Check sheet for the modelled part. Datum: model origin and axes. Units: mm. Face numbers are marked on the shaded views. Round coordinates to 2 decimals unless told otherwise and drop trailing zeros. Write each loop counter-clockwise with the first axis right and the second up, starting at its lowest first coordinate (ties: lowest second). Pieces come first, ordered by that corner, then holes.
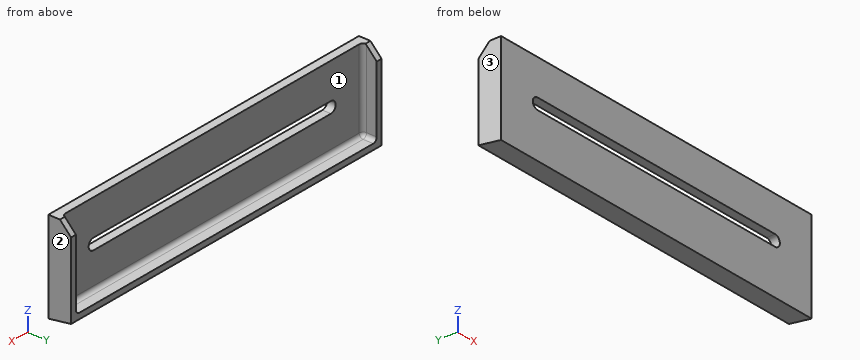
from build123d import *

# Parameters (mm, degrees)
SKETCH1_W           = 101.6
SKETCH1_H           = 25.4
BOSS_EXTRUDE1_DEPTH = 6.35
CUT_EXTRUDE2_DEPTH  = 101.6
SKETCH4_W           = 98.425
SKETCH4_H           = 22.79142
CUT_EXTRUDE3_DEPTH  = 3.96748
CUT_EXTRUDE6_DEPTH  = 2.54
CUT_EXTRUDE7_DEPTH  = 1.5875
CUT_EXTRUDE8_DEPTH  = 1.5875
FILLET1_R           = 1.12268


with BuildPart() as part:
    # Sketch1 → Boss-Extrude1 (new body)
    with BuildSketch(Plane(origin=(0, 0, 0), x_dir=(1, 0, 0), z_dir=(0, 1, 0))):
        Rectangle(SKETCH1_W, SKETCH1_H)
    extrude(amount=BOSS_EXTRUDE1_DEPTH)

    # Sketch2 → Cut-Extrude2 (cut)
    with BuildSketch(Plane.ZY.offset(50.8)):
        Polygon((-12.7, 0), (-11.67892, 6.35), (-12.7, 6.35), align=None)
    extrude(amount=-CUT_EXTRUDE2_DEPTH, mode=Mode.SUBTRACT)

    # Sketch4 → Cut-Extrude3 (cut)
    with BuildSketch(Plane(origin=(0, 6.35, 0), x_dir=(1, 0, 0), z_dir=(0, 1, 0))):
        with Locations((0, -1.30429)):
            Rectangle(SKETCH4_W, SKETCH4_H)
    extrude(amount=-CUT_EXTRUDE3_DEPTH, mode=Mode.SUBTRACT)

    # Sketch5 → Cut-Extrude6 (cut)
    with BuildSketch(Plane(origin=(0, 2.38252, 0), x_dir=(1, 0, 0), z_dir=(0, 1, 0))):
        with BuildLine():
            Line((-38.862, -2.818654725), (38.862, -2.818654725))
            ThreePointArc((38.862, -2.818654725), (40.410654725, -1.27), (38.862, 0.278654725))
            Line((38.862, 0.278654725), (-38.862, 0.278654725))
            ThreePointArc((-38.862, 0.278654725), (-40.410654725, -1.27), (-38.862, -2.818654725))
        make_face()
    extrude(amount=-CUT_EXTRUDE6_DEPTH, mode=Mode.SUBTRACT)

    # Sketch6 → Cut-Extrude7 (cut)
    with BuildSketch(Plane(origin=(-49.2125, 0, 0), x_dir=(0, 0, -1), z_dir=(1, 0, 0))):
        Polygon((-9.45896, 6.35), (-12.7, 3.22326), (-12.7, 6.35), align=None)
    extrude(amount=-CUT_EXTRUDE7_DEPTH, mode=Mode.SUBTRACT)

    # Sketch7 → Cut-Extrude8 (cut)
    with BuildSketch(Plane.ZY.offset(-49.2125)):
        Polygon((9.45896, 6.35), (12.7, 3.22326), (12.7, 6.35), align=None)
    extrude(amount=-CUT_EXTRUDE8_DEPTH, mode=Mode.SUBTRACT)

    # Fillet1
    fillet1_edges = [part.edges().sort_by_distance(p)[0] for p in [
        (49.2125, 4.36626, -10.09142),
        (49.2125, 2.38252, 1.30429),
        (-49.2125, 4.36626, -10.09142),
        (-49.2125, 2.38252, 1.30429),
        (0, 2.38252, -10.09142),
    ]]
    fillet(fillet1_edges, radius=FILLET1_R)


solid = part.part
1. Sectioned sample at D-D, the plane y = 4.5. Enter the section's corners in (x, z), plus the area to 3 significant figures.
2. Sectioned sample at B-B, the plane z = 1.27. Enter the section's corners in (x, y), plus the area to 3 significant figures.
3. Sectioned sample at C-C, the plane z = 8. Enter the section's corners in (x, y), plus the area to 3 significant figures.
4. Scan lines: line 1 along X through (y, z) = (5, 0.75); line 2 along Y through (x, z) = (37, -9); line 3 along X through (y, z) = (2.5, -2.25). Record each from-to range of solid material in increasing order.
5. Go/stop test with flat-tipped pins: pin 1 (2 mm diameter, centred on x = -35, y = 3.5, fed in from -Z); pin 2 (3 mm diameter, centred on x = 26.5, y = 2, fed in from -Z); pin 3 (0.9 mm diameter, centred on x = 10, y = 4.5, fed in from +Z). Record where each tip stops, or that it passes through.
6. Release check for a two-part mould opening along X. For the marked faces 1, 2 and 3 record: released by +X, released by -X, zero draft, split by the parting line, or undercut.
7. Sectioned sample at A-A, the plane x = 18. Enter the section's corners in (y, z).
Computed values:
1. outline: (-50.8, -11.98) - (50.8, -11.98) - (50.8, 11.38) - (49.21, 11.38) - (49.21, -8.97) arc R1.12 cw to (48.09, -10.09) - (-48.09, -10.09) arc R1.12 cw to (-49.21, -8.97) - (-49.21, 11.38) - (-50.8, 11.38) - close
1. area: 260 mm2
2. outline: (-50.8, 0) - (-40.41, 0) - (-40.41, 2.38) - (-48.09, 2.38) arc R1.12 cw to (-49.21, 3.51) - (-49.21, 6.35) - (-50.8, 6.35) - close; (40.41, 0) - (50.8, 0) - (50.8, 6.35) - (49.21, 6.35) - (49.21, 3.51) arc R1.12 cw to (48.09, 2.38) - (40.41, 2.38) - close
2. area: 62.6 mm2
3. outline: (-50.8, 0) - (50.8, 0) - (50.8, 6.35) - (49.21, 6.35) - (49.21, 3.51) arc R1.12 cw to (48.09, 2.38) - (-48.09, 2.38) arc R1.12 cw to (-49.21, 3.51) - (-49.21, 6.35) - (-50.8, 6.35) - close
3. area: 255 mm2
4. line 1: x = -50.8 to -49.21, 49.21 to 50.8
4. line 2: y = 0 to 2.38
4. line 3: x = -50.8 to -48.59, 48.59 to 50.8
5. pin 1: stops at z = -12.3
5. pin 2: stops at z = -12.62
5. pin 3: stops at z = -10.09
6. face 1: undercut
6. face 2: released by +X
6. face 3: released by -X
7. outline: (0, -12.7) - (6.35, -11.68) - (6.35, -10.09) - (3.51, -10.09) arc R1.12 cw to (2.38, -8.97) - (2.38, -0.28) - (0, -0.28) - close; (0, 2.82) - (2.38, 2.82) - (2.38, 12.7) - (0, 12.7) - close
